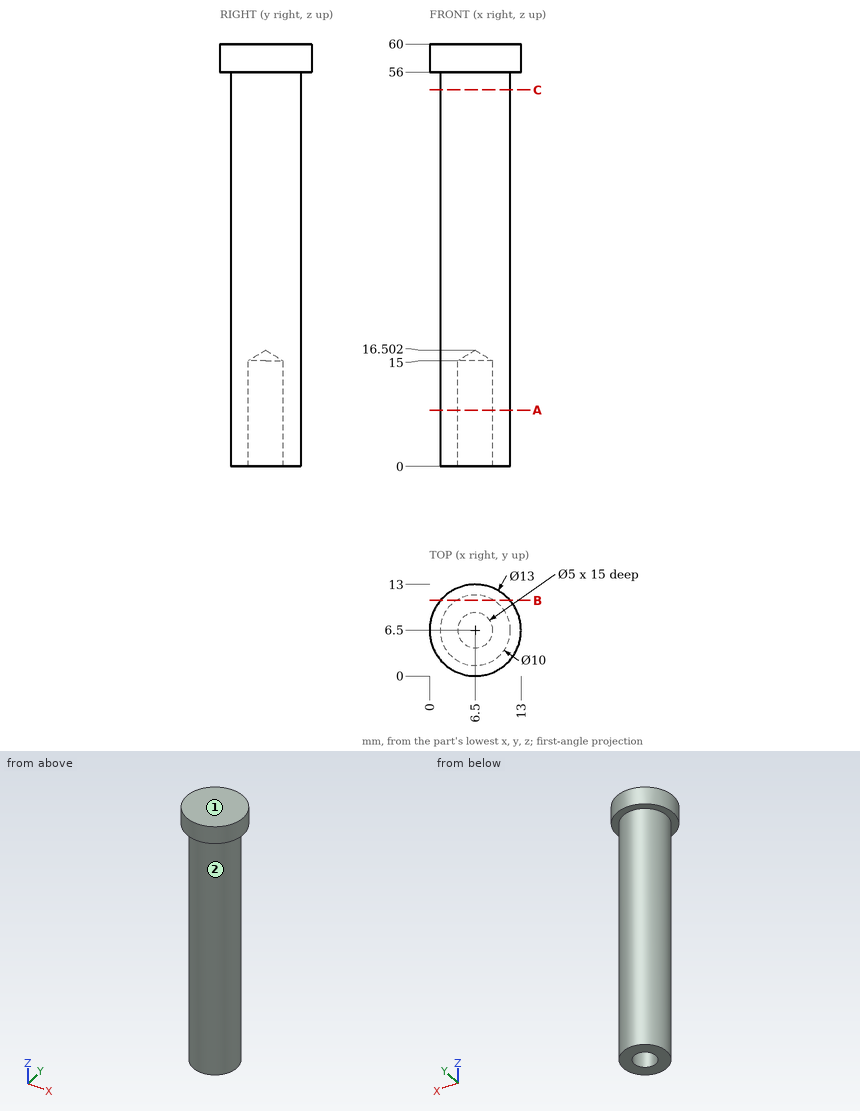
Verification items for this drawing (mm, ordinates from the low corner). A direction names the side the tool comes from. Round coordinates to 2 decimals unless told otherwise and drop trailing zeros. Write each loop counter-clockwise with the first axis right and the second up, starting at its lowest first coordinate (ties: lowest second). Pieces come first, ordered by that corner, then holes. Notation, with made-up numbers: (37, 60.5) - (84, 60.5) arc R23 cw to (84, 84.5) - close; hole circle Ø1 at (76, -12.5). An arc over 180 degrees is marked (long way). One line per item, written item: value.
1. Depth check by flat-ended pin: pin 1 Ø1.5 at (y, z) = (4, 31.5) entering from +X; pin 2 Ø4 at (y, z) = (5.5, 15) entering from -X; pin 3 Ø4.5 at (x, y) = (6.5, 6.5) entering from -Z. Enter the tip coordinate at first touch or a pass-through.
The answers:
pin 1: stops at x = 11.18
pin 2: stops at x = 1.5
pin 3: stops at z = 15.15
2. Cross-section at B-B on y = 10.75. Record the boundary of the cut face in (x, z).
The answers:
outline: (1.58, 56) - (3.87, 56) - (3.87, 0) - (9.13, 0) - (9.13, 56) - (11.42, 56) - (11.42, 60) - (1.58, 60) - close
3. Scan lines: L1, parallel to Y at x = 6.5, z = 3.5; L2, parallel to Z at x = 10.5, y = 2; L3, parallel to Y at x = 5.25, z = 9 (1 decimal). Record each from-to range of solid material in increasing order.
The answers:
L1: y = 1.5 to 4, 9 to 11.5
L2: z = 56 to 60
L3: y = 1.7 to 4.3, 8.7 to 11.3
4. Cross-section at A-A on z = 8. Record the boundary of the cut face in (x, y).
The answers:
outline: circle Ø10 at (6.5, 6.5); hole circle Ø5 at (6.5, 6.5)
5. Set-up check for the marked faces 1 and 2: record each of +Z, -Z, +X, -X, +Y, -Y from which the full face is reachable in a straight line by a thin tool's end or side.
The answers:
face 1: +Z, +X, -X, +Y, -Y
face 2: -Z
6. Cross-section at C-C on z = 53.5. Record the boundary of the cut face in (x, y).
The answers:
outline: circle Ø10 at (6.5, 6.5)
